Part model, mm, in its own coordinate system. A direction names the side the tool comes from. Round coordinates to 2 decimals unless told otherwise and drop trailing zeros. Loops run counter-clockwise (first coordinate to the right, second up) from the corner with the lowest first, then second, coordinate; pieces in that order, holes last.
(1) Cut at A-A on z = 0. List the corners of the cut face in (x, y), then the cut area to 3 significant figures.
(2) Cut at C-C on y = 129.5. List the corners of the cut face in (x, z).
(3) Cut at D-D on y = 68. List the corners of the cut face in (x, z), then the cut area to 3 significant figures.
(4) Probe probe 1 along Y at (x, z) = (223.5, -5.5); probe 2 along X at (y, z) = (64.5, 0.5); probe 3 along X at (y, z) = (4.5, 8.5). List the from-to ranges inside material, lowest first.
(5) Tool access for faces 1 (the face through (0, 0, 0)), 2 (the face through (250, 200, 0)), 3 (the face through (264.872, -49.3, 1.953)): list every direction of +Z, -Z, +X, -X, +Y, -Y with a clear straight run to the whole face (end or side of a thin tool).
(6) Flat gauge pins, fed straight in: pin 1 (5 mm diameter, centred on x = 178, y = 113, fed in from +Z); pin 2 (3 mm diameter, centred on x = 9.5, z = 4.5, fed in from +Y); pin 3 (1.5 mm diameter, centred on y = -66.5, z = 11.5, fed in from -X); pin 4 (6 mm diameter, centred on x = 12, z = -7.5, fed in from -Y). Where does each tip first touch, or does it go through?
(7) Cut at B-B on x = 58.5. List the corners of the cut face in (y, z).
from build123d import *
from build123d.topology import SkipClean

# Parameters (mm, degrees)
SKETCH1_R           = 20
BOSS_EXTRUDE1_DEPTH = 10
BOSS_EXTRUDE2_DEPTH = 100
BOSS_EXTRUDE3_START = 10
SKETCH3_R           = 20
BOSS_EXTRUDE3_DEPTH = 10
SKETCH6_R           = 20
BOSS_EXTRUDE5_DEPTH = 90
SKETCH9_R           = 15
BOSS_EXTRUDE6_DEPTH = 100


with BuildPart() as part:
    # Sketch1 → Boss-Extrude1 (new body)
    with BuildSketch(Plane(origin=(0, 0, 0), x_dir=(1, 0, 0), z_dir=(0, 1, 0))):
        with Locations(Location((0, 0, 0), (0, 0, 270))):
            Circle(SKETCH1_R)
    extrude(amount=BOSS_EXTRUDE1_DEPTH)

    # Sketch2 → Boss-Extrude2 (add)
    with BuildSketch(Plane(origin=(0, 10, 0), x_dir=(1, 0, 0), z_dir=(0, 1, 0))):
        with BuildLine():
            Line((0, -20), (250, -20))
            ThreePointArc((250, -20), (270, 0), (250, 20))
            Line((250, 20), (0, 20))
            ThreePointArc((0, 20), (-20, 0), (0, -20))
        make_face()
    extrude(amount=BOSS_EXTRUDE2_DEPTH)

    # Sketch3 → Boss-Extrude3 (add)
    with SkipClean():  # the faces are left unmerged after this step: merging them gives an invalid solid
        with BuildSketch(Plane.XZ.offset(-10).offset(BOSS_EXTRUDE3_START)):
            with Locations(Location((250, 0, 0), (0, 0, 270))):
                Circle(SKETCH3_R)
        extrude(amount=-BOSS_EXTRUDE3_DEPTH)

    # Sketch6 → Boss-Extrude5 (add)
    with BuildSketch(Plane(origin=(0, 110, 0), x_dir=(1, 0, 0), z_dir=(0, 1, 0))):
        with Locations(Location((250, 0, 0), (0, 0, 90))):
            Circle(SKETCH6_R)
    extrude(amount=BOSS_EXTRUDE5_DEPTH)

    # Sketch9 → Boss-Extrude6 (add)
    with BuildSketch(Plane.XZ):
        with Locations(Location((250, 0, 0), (0, 0, 270))):
            Circle(SKETCH9_R)
    extrude(amount=BOSS_EXTRUDE6_DEPTH)


solid = part.part
Final values:
1. outline: (-20, 0) - (20, 0) - (20, 10) - (230, 10) - (230, 0) - (235, 0) - (235, -100) - (265, -100) - (265, 0) - (270, 0) - (270, 200) - (230, 200) - (230, 110) - (-20, 110) - close
1. area: 36,400 mm2
2. outline: circle Ø40 at (250, 0)
3. outline: (0, -20) - (250, -20) arc R20 ccw to (250, 20) - (0, 20) arc R20 ccw to start
3. area: 11,300 mm2
4. probe 1: y = 10 to 110
4. probe 2: x = -19.99 to 269.99
4. probe 3: x = -18.1 to 18.1, 231.9 to 268.1
5. face 1: +Z, -Z, -X, -Y
5. face 2: +Z, -Z, +X, -X, +Y
5. face 3: -Y
6. pin 1: passes through
6. pin 2: stops at y = 110
6. pin 3: stops at x = 239.54
6. pin 4: stops at y = 0
7. outline: (10, -20) - (110, -20) - (110, 20) - (10, 20) - close
